from build123d import *

# Parameters (mm, degrees)
RESSALTO_EXTRUS_O1_DEPTH   = 66
CORTE_EXTRUS_O1_DEPTH      = 53.5
CORTE_EXTRUS_O2_DEPTH      = 63
CORTE_EXTRUS_O3_DEPTH      = 75.455375226
CORTE_EXTRUS_O3_DEPTH_BACK = 75.455375226
CORTE_EXTRUS_O4_DEPTH      = 61.725636267
CORTE_EXTRUS_O4_DEPTH_BACK = 61.725636267
ESBO_O5_W                  = 2
ESBO_O5_H                  = 8
CORTE_EXTRUS_O5_DEPTH      = 47
CORTE_EXTRUS_O7_DEPTH      = 10


with BuildPart() as part:
    # Esboço1 → Ressalto-extrusão1 (new body)
    with BuildSketch(Plane(origin=(0, 0, 0), x_dir=(1, 0, 0), z_dir=(0, 1, 0))):
        with BuildLine():
            Line((-13.376104721, 16.054091922), (-22.876104721, -1.295908078))
            ThreePointArc((-22.876104721, -1.295908078), (-22.619735169, -16.393998269), (-9.5, -23.87))
            Line((-9.5, -23.87), (9.5, -23.87))
            ThreePointArc((9.5, -23.87), (22.619735169, -16.393998269), (22.876104721, -1.295908078))
            Line((22.876104721, -1.295908078), (13.376104721, 16.054091922))
            ThreePointArc((13.376104721, 16.054091922), (0, 23.98), (-13.376104721, 16.054091922))
        make_face()
    extrude(amount=RESSALTO_EXTRUS_O1_DEPTH)

    # Esboço2 → Corte-extrusão1 (cut)
    with BuildSketch(Plane(origin=(0, 66, 0), x_dir=(1, 0, 0), z_dir=(0, 1, 0))):
        with BuildLine():
            Line((-18.929057426, -3.45711553), (-9.429057426, 13.89288447))
            ThreePointArc((-9.429057426, 13.89288447), (0, 19.48), (9.429057426, 13.89288447))
            Line((9.429057426, 13.89288447), (18.929057426, -3.45711553))
            ThreePointArc((18.929057426, -3.45711553), (18.748337906, -14.100031567), (9.5, -19.37))
            Line((9.5, -19.37), (-9.5, -19.37))
            ThreePointArc((-9.5, -19.37), (-18.748337906, -14.100031567), (-18.929057426, -3.45711553))
        make_face()
    extrude(amount=-CORTE_EXTRUS_O1_DEPTH, mode=Mode.SUBTRACT)

    # Esboço3 → Corte-extrusão2 (cut)
    with BuildSketch(Plane(origin=(0, 66, 0), x_dir=(1, 0, 0), z_dir=(0, 1, 0))):
        with BuildLine():
            Line((0, -3.37), (18.88135728, -3.37))
            Line((18.88135728, -3.37), (9.429057426, 13.89288447))
            ThreePointArc((9.429057426, 13.89288447), (0, 19.48), (-9.429057426, 13.89288447))
            Line((-9.429057426, 13.89288447), (-18.88135728, -3.37))
            Line((-18.88135728, -3.37), (0, -3.37))
        make_face()
    extrude(amount=-CORTE_EXTRUS_O2_DEPTH, mode=Mode.SUBTRACT)

    # Esboço4 → Corte-extrusão3 (cut, two sides: drawn at the far end of the back side and taken through both)
    with BuildSketch(Plane(origin=(0, 0, 0), x_dir=(0, 0, -1), z_dir=(1, 0, 0)).offset(-CORTE_EXTRUS_O3_DEPTH_BACK)):
        Polygon((-8.37, 50), (35.337515561, 50), (33.498972566, 68.632714226), (-19.37, 68.632714226), (-19.37, 66), align=None)
    extrude(amount=CORTE_EXTRUS_O3_DEPTH + CORTE_EXTRUS_O3_DEPTH_BACK, mode=Mode.SUBTRACT)

    # Esboço5 → Corte-extrusão4 (cut, two sides: drawn at the far end of the back side and taken through both)
    with BuildSketch(Plane(origin=(0, 50, 0), x_dir=(1, 0, 0), z_dir=(0, 1, 0)).offset(-CORTE_EXTRUS_O4_DEPTH_BACK)):
        with Locations((6, 7.13)):
            Rectangle(ESBO_O5_W, ESBO_O5_H)
        with Locations((-6, 7.13)):
            Rectangle(ESBO_O5_W, ESBO_O5_H)
    extrude(amount=CORTE_EXTRUS_O4_DEPTH + CORTE_EXTRUS_O4_DEPTH_BACK, mode=Mode.SUBTRACT)

    # Esboço6 → Corte-extrusão5 (cut)
    with BuildSketch(Plane(origin=(0, 50, 0), x_dir=(1, 0, 0), z_dir=(0, 1, 0))):
        Polygon((0, 12.98), (14, 12.98), (14, 7.98), (-14, 7.98), (-14, 12.98), align=None)
    extrude(amount=-CORTE_EXTRUS_O5_DEPTH, mode=Mode.SUBTRACT)

    # Esboço7 → Corte-extrusão7 (cut)
    with BuildSketch(Plane(origin=(0, 50, 0), x_dir=(1, 0, 0), z_dir=(0, 1, 0))):
        Polygon((0, 3.70102494), (16.346068598, 10.63), (21.821572921, 0.63), (0, -8.62), (-21.821572921, 0.63), (-16.346068598, 10.63), align=None)
    extrude(amount=-CORTE_EXTRUS_O7_DEPTH, mode=Mode.SUBTRACT)


solid = part.part
For this review, take the finished solid that the model builds, in its own axes (mm). A direction names the side the tool comes from. Round coordinates to 2 decimals unless told otherwise and drop trailing zeros. Write each loop counter-clockwise with the first axis right and the second up, starting at its lowest first coordinate (ties: lowest second). Pieces come first, ordered by that corner, then holes. Notation, with made-up numbers: (17, -28) - (71, -28) arc R23 ccw to (71, -12) - close; hole circle Ø1 at (71.25, 71). An arc over 180 degrees is marked (long way). Use a Markdown table: item, result.
Q1. We need section A-A (y = 31). Give the boundary of the cut face in (x, z), plus the area to 3 significant figures.
Derived:
| item | result |
|---|---|
| outline | (-22.88, 1.3) - (-13.38, -16.05) arc R15.25 ccw to (13.38, -16.05) - (22.88, 1.3) arc R15.25 ccw to (9.5, 23.87) - (-9.5, 23.87) arc R15.25 ccw to start; hole (-18.93, 3.46) - (-12.67, -7.98) - (-14, -7.98) - (-14, -12.98) - (-9.93, -12.98) - (-9.43, -13.89) arc R10.75 ccw to (9.43, -13.89) - (9.93, -12.98) - (14, -12.98) - (14, -7.98) - (12.67, -7.98) - (18.93, 3.46) arc R10.75 ccw to (9.5, 19.37) - (-9.5, 19.37) arc R10.75 ccw to start |
| area | 604 mm2 |
Q2. Wall thickness on line 1 along Z through (x, y) = (-10, 3.5); line 2 along Z through (x, y) = (-1.5, 20.5); line 3 along Y through (x, z) = (9.5, -5): over which ranges is each line inside the solid? List them lowest first.
Derived:
| item | result |
|---|---|
| line 1 | z = -20.24 to -12.98, 3.37 to 23.86 |
| line 2 | z = -23.91 to -19.37, 19.37 to 23.87 |
| line 3 | y = 0 to 3 |
Q3. Clearance check with flat-ended pins moving along their axes: pin 1 (2.5 mm diameter, centred on x = 17, z = -6, fed in from +Y); pin 2 (10 mm diameter, centred on x = -13.5, y = 50, fed in from -Z); pin 3 (1 mm diameter, centred on y = 7, z = 6, fed in from -X). State where each tip first meets the part, or that it passes through.
Derived:
| item | result |
|---|---|
| pin 1 | stops at y = 40 |
| pin 2 | stops at z = -21.39 |
| pin 3 | stops at x = -24.6 |
Q4. We need section C-C (x = 0). Give the boundary of the cut face in (y, z), plus the area to 3 significant figures.
Derived:
| item | result |
|---|---|
| outline | (0, -23.98) - (50, -23.98) - (50, -19.48) - (3, -19.48) - (3, 3.37) - (12.5, 3.37) - (12.5, 19.37) - (66, 19.37) - (66, 23.87) - (0, 23.87) - close |
| area | 791 mm2 |
Q5. We need section D-D (z = -5). Give the boundary of the cut face in (x, y).
Derived:
| item | result |
|---|---|
| outline | (-19.43, 0) - (-7, 0) - (-7, 3) - (-14.3, 3) - (-14.3, 40) - (-19.43, 40) - close; (-5, 0) - (5, 0) - (5, 3) - (-5, 3) - close; (7, 0) - (19.43, 0) - (19.43, 40) - (14.3, 40) - (14.3, 3) - (7, 3) - close |
Q6. The part is to be moulded in two halves that separate along Z. For faces 6 (the flat face through (-17, 40, -5)), 7 (the cylindrical face through (22.51, 32.54, 16.58)), 8 (the flat face through (20.478, 58.63, 14.303)), say which applies: pulls with the +Z half, pulls with the -Z half, needs draft (parallel to the pull), parting line crosses it, or undercut.
Derived:
| item | result |
|---|---|
| face 6 | undercut |
| face 7 | parting line crosses it |
| face 8 | pulls with the -Z half |
Q7. Machinability: for faces 1 (the flat face through (0, 0, 5)), 2 (the flat face through (18.19, 24.65, -7.26)), 3 (the flat face through (-19.71, 45.07, 0.265)), 4 (the flat face through (14, 27, -11)), 5 (the flat face through (7, 1, -7)), which of the approach directions +Z, -Z, +X, -X, +Y, -Y give a long, thin tool a straight path to every point of the face, cutting with its end or side? Answer none if there is none.
Derived:
| item | result |
|---|---|
| face 1 | +Z, -Z, +X, -X, -Y |
| face 2 | -Z, +X, +Y, -Y |
| face 3 | -Z, +Y |
| face 4 | +Y |
| face 5 | +Y, -Y |
Q8. We need section B-B (y = 49). Give the boundary of the cut face in (x, z).
Derived:
| item | result |
|---|---|
| outline | (-22.88, 1.3) - (-21.82, -0.63) - (-17.66, 1.14) - (-18.93, 3.46) arc R10.75 cw to (-9.5, 19.37) - (9.5, 19.37) arc R10.75 cw to (18.93, 3.46) - (17.66, 1.14) - (21.82, -0.63) - (22.88, 1.3) arc R15.25 ccw to (9.5, 23.87) - (-9.5, 23.87) arc R15.25 ccw to start; (-16.35, -10.63) - (-13.38, -16.05) arc R15.25 ccw to (13.38, -16.05) - (16.35, -10.63) - (14, -9.64) - (14, -12.98) - (9.93, -12.98) - (9.43, -13.89) arc R10.75 cw to (-9.43, -13.89) - (-9.93, -12.98) - (-14, -12.98) - (-14, -9.64) - close |
